Job drawing, mm, ordinate dimensions from the low corner. One solid piece. A direction names the side the tool comes from. Coordinates: 2 decimals unless noted, no trailing zeros. Write each loop counter-clockwise with the first axis right and the second up, starting at its lowest first coordinate (ties: lowest second). Pieces come first, ordered by that corner, then holes. Notation, with made-up numbers: (31.5, 54) -> (77.5, 54) arc R8 ccw to (77.5, 66) -> close; hole circle Ø6 at (51, 0). An arc over 180 degrees is marked (long way). One line per question, with ' | ' between items. Start each with the question number.
Item 1: Probe probe 1 along Z at (x, y) = (90, 69.5); probe 2 along Y at (x, z) = (52, 290); probe 3 along X at (y, z) = (47, 163). List the from-to ranges inside material, lowest first. Write a range as [from, to].
Item 2: Saw through at D-D (y = 88). List the corners of the cut face in (x, z), and give its area (3 significant figures).
Item 3: Pin check, flat tips, straight feed: pin 1 (3 mm diameter, centred on y = 80, z = 214, fed in from -X); pin 2 (5 mm diameter, centred on x = 82, y = 35, fed in from +Z); pin 3 (1.5 mm diameter, centred on x = 77, y = 80.5, fed in from -Z). Stop position of each tip, or through.
Item 4: Saw through at C-C (z = 293.5). List the corners of the cut face in (x, y).
Item 5: 3-axis set-ups, long thin cutter, end or side, ignore diameter. For the marked faces 1 and 2: which of +Z, -Z, +X, -X, +Y, -Y reach the whole face in a straight line?
Item 6: Saw through at A-A (x = 50). List the corners of the cut face in (y, z).
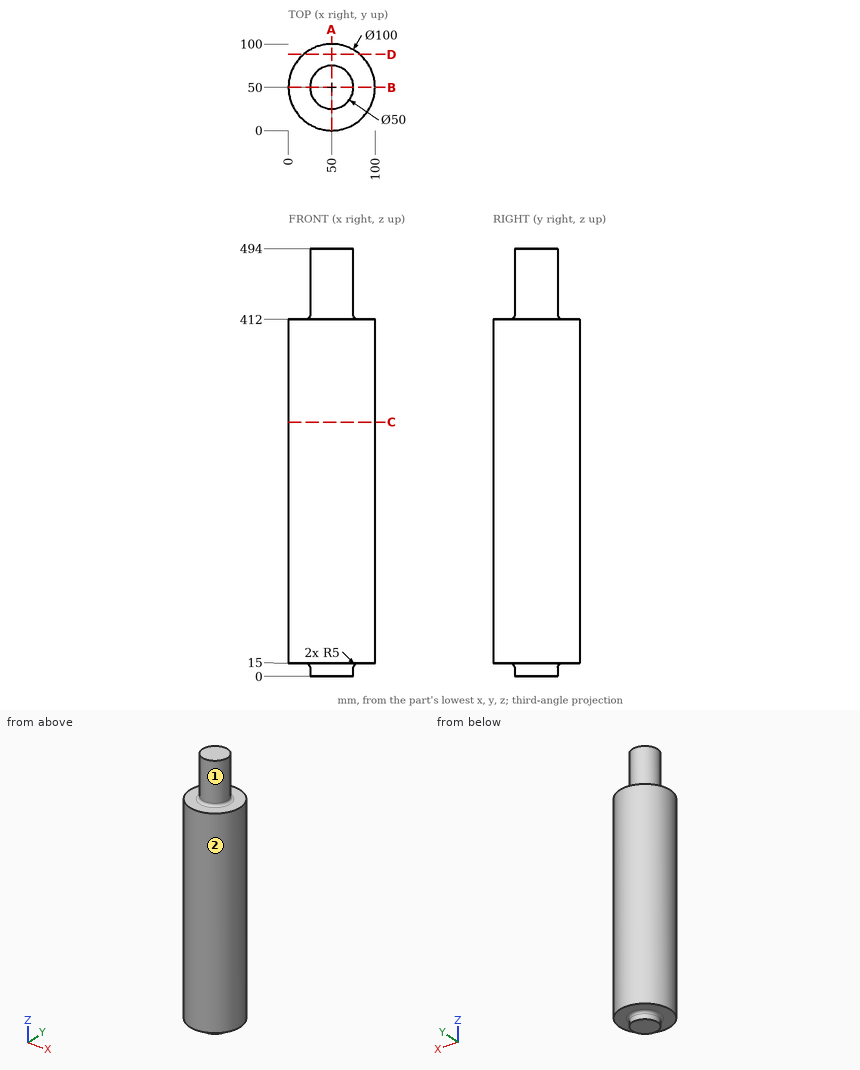
From the geometry:
1) probe 1: [15, 412] | probe 2: [0.04, 99.96] | probe 3: [0.09, 99.91]
2) outline: (17.5, 15) -> (82.5, 15) -> (82.5, 412) -> (17.5, 412) -> close | area: 25,800 mm2
3) pin 1: x = 8.92 | pin 2: z = 412 | pin 3: z = 15
4) outline: circle Ø100 at (50, 50)
5) face 1: +Z | face 2: +Z, -Z
6) outline: (0, 15) -> (20, 15) arc R5 cw to (25, 10) -> (25, 0) -> (75, 0) -> (75, 10) arc R5 cw to (80, 15) -> (100, 15) -> (100, 412) -> (80, 412) arc R5 cw to (75, 417) -> (75, 494) -> (25, 494) -> (25, 417) arc R5 cw to (20, 412) -> (0, 412) -> close
